```python
from build123d import *

# Parameters (mm, degrees)
PAD_DEPTH = 495


with BuildPart() as part:
    # Sketch → Pad (new body)
    with BuildSketch(Plane.XZ):
        with BuildLine():
            Line((0, 3), (165, 3))
            Line((165, 3), (165, 0))
            Line((165, 0), (0, 0))
            ThreePointArc((0, 0), (-10.606602, -4.393398), (-15, -15))
            Line((-15, -15), (-15, -125))
            Line((-15, -125), (-18, -125))
            Line((-18, -125), (-18, -15))
            ThreePointArc((0, 3), (-12.727922, -2.272078), (-18, -15))
        make_face()
    extrude(amount=PAD_DEPTH)


solid = part.part
```
The listing builds one solid part. Answer for the finished solid, in the listing's coordinates (mm). A direction names the side the tool comes from. Give positions to 0.01 mm unless a question says otherwise; leave off trailing zeros. Order: outer loops, then holes, each group sorted by start corner. A loop starts at its lowest first (then second) coordinate and runs counter-clockwise, first axis right, second up. Notation, with made-up numbers: (36.5, 5) -> (94.5, 5) arc R22 cw to (94.5, 41) -> close; hole circle Ø1 at (-16.5, 87.25). An arc over 180 degrees is marked (long way). Answer as a JSON object with one key per item and string values. Group by question number.
Item 1: Consider L1, parallel to X at y = -103, z = -69; L2, parallel to Z at x = 18.5, y = -60.5; L3, parallel to X at y = -263.5, z = -6. Determine where each line is inside the solid, lowest interval first. Write a range as from..to.
Item 2: Flat-ended cylindrical pins translate along their axes: pin 1 (1.5 mm diameter, centred on y = -129, z = -62, fed in from +X); pin 2 (3 mm diameter, centred on x = 79.5, y = -153.5, fed in from -Z); pin 3 (4 mm diameter, centred on y = -266, z = -13, fed in from +X). Find the tip coordinate at first contact, or state that the pin passes through.
Item 3: The part is cut by section A-A on y = -328.5. Write down the section's boundary in (x, z).
Item 4: The part is cut by section B-B on x = 143. Write down the section's boundary in (y, z).
Item 5: A tool of negligible diameter and unlimited length cuts with its end or side. For faces 1 (the flat face through (-15, -244, -69)), 2 (the flat face through (81, -244, 3)), from which of +Z, -Z, +X, -X, +Y, -Y can it reach the whole face along a straight path? Write none if from no direction.
Item 6: The part is cut by section C-C on z = -62.5. Write down the section's boundary in (x, y), and give its area (4 significant figures).
Result set:
{
 "1": {"L1": "-18..-15", "L2": "0..3", "L3": "-15.59..-12"},
 "2": {"pin 1": "x = -15", "pin 2": "z = 0", "pin 3": "x = -14.46"},
 "3": {"outline": "(-18, -125) -> (-15, -125) -> (-15, -15) arc R15 cw to (0, 0) -> (165, 0) -> (165, 3) -> (0, 3) arc R18 ccw to (-18, -15) -> close"},
 "4": {"outline": "(-495, 0) -> (0, 0) -> (0, 3) -> (-495, 3) -> close"},
 "5": {"face 1": "-Z, +X, +Y, -Y", "face 2": "+Z, +X, -X, +Y, -Y"},
 "6": {"outline": "(-18, -495) -> (-15, -495) -> (-15, 0) -> (-18, 0) -> close", "area": "1,485 mm²"}
}
